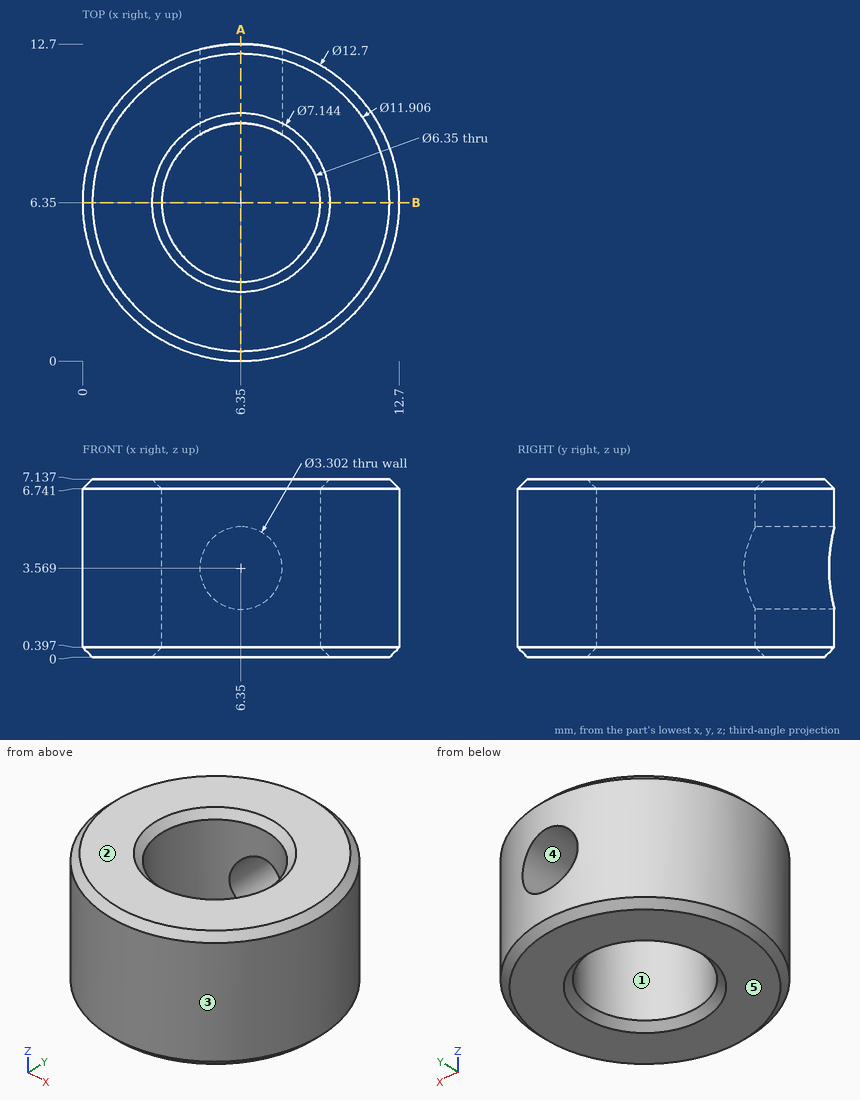
Here's the drawing with two shaded views (mm, measured from the low corner). I have some questions. A direction names the side the tool comes from. Give positions to 0.01 mm unless a question says otherwise; leave off trailing zeros. Loops run counter-clockwise (first coordinate to the right, second up) from the corner with the lowest first, then second, coordinate; pieces in that order, holes last. Notation, with made-up numbers: (55, -14) - (95, -14) arc R38 ccw to (95, 25) - close; hole circle Ø1 at (-11.5, 86). An arc over 180 degrees is marked (long way). Return JSON: item names as keys, results as strings.
1. We'd pull the mould along X, two halves only. Please class the marked faces 1, 2 and 3: +X half, -X half, draft (parallel to the pull), parting line (faces both ways), or undercut.
Output values:
{"face 1": "undercut", "face 2": "draft", "face 3": "parting line"}
2. If I drill on line 1 (Y direction, x = 6.35, z = 5.75) (1 decimal); line 2 (Y direction, x = 6.35, z = 3.5) (1 decimal); line 3 (X direction, y = 4.75, z = 5) (1 decimal), over which ranges is the centre line in solid material (lowest first)?
Output values:
{"line 1": "y = 0 to 3.2, 9.5 to 12.7", "line 2": "y = 0 to 3.2", "line 3": "x = 0.2 to 3.6, 9.1 to 12.5"}
3. I'm going to push flat-ended pins straight in: pin 1 Ø5.5 at (x, y) = (6.35, 6.35) entering from +Z; pin 2 Ø3 at (x, z) = (10.5, 2.5) entering from -Y; pin 3 Ø1 at (y, z) = (5, 6) entering from +X. Where does each tip first touch, or does it pass through?
Output values:
{"pin 1": "passes through", "pin 2": "stops at y = 0.58", "pin 3": "stops at x = 12.64"}
4. For the marked faces 4 and 5, which set-ups out of +Z, -Z, +X, -X, +Y, -Y let a thin tool reach every point of the face, with its end or its side?
Output values:
{"face 4": "+Y", "face 5": "-Z, +X, -X, +Y, -Y"}
5. I want a section at A-A on x = 6.35. Please give me the cut outline in (y, z) (1 decimal), and give its area (3 significant figures).
Output values:
{"outline": "(0, 0.4) - (0.4, 0) - (2.8, 0) - (3.2, 0.4) - (3.2, 6.7) - (2.8, 7.1) - (0.4, 7.1) - (0, 6.7) - close; (9.5, 0.4) - (9.9, 0) - (12.3, 0) - (12.7, 0.4) - (12.7, 1.9) - (9.5, 1.9) - close; (9.5, 5.2) - (12.7, 5.2) - (12.7, 6.7) - (12.3, 7.1) - (9.9, 7.1) - (9.5, 6.7) - close", "area": "34.2 mm²"}
6. I want a section at B-B on y = 6.35. Please give me the cut outline in (x, z) (1 decimal), and give its area (3 significant figures).
Output values:
{"outline": "(0, 0.4) - (0.4, 0) - (2.8, 0) - (3.2, 0.4) - (3.2, 6.7) - (2.8, 7.1) - (0.4, 7.1) - (0, 6.7) - close; (9.5, 0.4) - (9.9, 0) - (12.3, 0) - (12.7, 0.4) - (12.7, 6.7) - (12.3, 7.1) - (9.9, 7.1) - (9.5, 6.7) - close", "area": "44.7 mm²"}
